```python
from build123d import *

# Parameters (mm, degrees)
F0_R     = 1.25
F1_DEPTH = 5
F2_DEPTH = 6
F3_R     = 3.5
F4_DEPTH = 2
F5_R     = 3.5
F6_DEPTH = 2
F7_R     = 0.99999


# Not quite as in the source:
# - a fillet or chamfer is up to 0.001 mm smaller than in the source, because OpenCascade refuses the exact size


with BuildPart() as f1:
    # F0 (on Top) → F1 (new body)
    with BuildSketch(Plane.XY):
        with BuildLine():
            ThreePointArc((-24.6972243623, -3), (-23.4537141687, -1.7234101758), (-23, 0))
            ThreePointArc((-23, 0), (-23.4537141687, 1.7234101758), (-24.6972243623, 3))
            ThreePointArc((-24.6972243623, 3), (-30, 0), (-24.6972243623, -3))
        make_face()
        with Locations((-26.5, 0)):
            Circle(F0_R, mode=Mode.SUBTRACT)
    extrude(amount=F1_DEPTH)



with BuildPart() as f1b:
    # F0 (on Top) → F1, piece 2 (new body)
    with BuildSketch(Plane.XY):
        with BuildLine():
            ThreePointArc((30, 0), (28.2234101758, 3.0462858313), (24.6972243623, 3))
            ThreePointArc((24.6972243623, 3), (23, 0), (24.6972243623, -3))
            ThreePointArc((24.6972243623, -3), (28.2234101758, -3.0462858313), (30, 0))
        make_face()
        with Locations((26.5, 0)):
            Circle(F0_R, mode=Mode.SUBTRACT)
    extrude(amount=F1_DEPTH)


with BuildPart() as f1_1:
    add(f1.part)

    add(f1b.part)  # F2 merges F1b
    # F0 (on Top) → F2 (join)
    with BuildSketch(Plane.XY):
        with BuildLine():
            ThreePointArc((-24.6972243623, 3), (-23.4537141687, 1.7234101758), (-23, 0))
            ThreePointArc((-23, 0), (-23.4537141687, -1.7234101758), (-24.6972243623, -3))
            Line((-24.6972243623, -3), (24.6972243623, -3))
            ThreePointArc((24.6972243623, -3), (23, 0), (24.6972243623, 3))
            Line((24.6972243623, 3), (-24.6972243623, 3))
        make_face()
    extrude(amount=F2_DEPTH)

    # F3 (on face) → F4 (join)
    with BuildSketch(Plane.XY.offset(5)):
        with Locations((-26.5, 0)):
            Circle(F3_R)
    extrude(amount=F4_DEPTH)

    # F5 (on face) → F6 (join)
    with BuildSketch(Plane.XY.offset(5)):
        with Locations((26.5, 0)):
            Circle(F5_R)
    extrude(amount=F6_DEPTH)

    # F7 (radius 1 in the source; OpenCascade refuses exactly that, so slightly less here)
    f7_edges = [f1_1.edges().sort_by_distance(p)[0] for p in [
        (0, 3, 6),
        (0, -3, 6),
        (23, 0, 7),
        (-30, 0, 7),
    ]]
    fillet(f7_edges, radius=F7_R)


solid = f1_1.part
```
CAD build for the part. Positions are in the model's coordinates, mm. A direction names the side the tool comes from. Give positions to 0.01 mm unless a question says otherwise; leave off trailing zeros. Order: outer loops, then holes, each group sorted by start corner. A loop starts at its lowest first (then second) coordinate and runs counter-clockwise, first axis right, second up. Notation, with made-up numbers: M 71,-4 L 101,-4 A29 cw 101,29 Z; hole C -5.75,-25 d4. An arc over 180 degrees is marked long. Put each result on its own line as item: value. Start each with the question number.
(1) Saw through at A-A, the plane x = -26.5. Write the cut outline in (y, z).
(2) Flat gauge pins, fed straight in: pin 1 Ø1.5 at (y, z) = (2.5, 1.5) entering from -X; pin 2 Ø0.8 at (x, y) = (27, 0.5) entering from -Z; pin 3 Ø1.5 at (x, z) = (-14, 3.5) entering from +Y. Where does each tip first touch, or does it go through?
(3) Drill centre lines: line 1 along Y through (x, z) = (-26.5, 1.5); line 2 along Z through (x, y) = (0, 1.25); line 3 along Y through (x, z) = (14.5, 3.25). Where is each one in solid material? Low to high.
(4) Saw through at B-B, the plane z = 3.75. Write the cut outline in (x, y).
(5) Which spindle directions (+Z, -Z, +X, -X, +Y, -Y) get a long thin tool onto all of the face, cutting with end or side? Do faces 4 (the cylindrical face through (-25.345, -0.479, 2.465)), 5 (the flat face through (0, 3, 2)), 6 (the flat face through (-27, 0, 7)), 7 (the cylindrical face through (0.346, -2.699, 5.715)), 8 (the flat face through (0, -3, 2)). Say none if no direction does.
(6) Mould opens along X. For faces 1 (the flat face through (26, 0, 5)), 2 (the flat face through (0, 0, 0)), 3 (the cylindrical face through (-0.346, 2.715, 5.699)) say: +X half, -X half, draft (parallel to the pull), parting line (faces both ways), or undercut.
Check result:
1. outline: M -3.5,0 L -1.25,0 L -1.25,5 L 1.25,5 L 1.25,0 L 3.5,0 L 3.5,6 A1 ccw 2.5,7 L -2.5,7 A1 ccw -3.5,6 Z
2. pin 1: stops at x = -29.53
2. pin 2: stops at z = 5
2. pin 3: stops at y = 3
3. line 1: y = -3.5 to -1.25, 1.25 to 3.5
3. line 2: z = 0 to 6
3. line 3: y = -3 to 3
4. outline: M -24.7,-3 L 24.7,-3 A3.5 ccw long 24.7,3 L -24.7,3 A3.5 ccw long Z; hole C -26.5,0 d2.5; hole C 26.5,0 d2.5
5. face 4: -Z
5. face 5: +Z, -Z, +Y
5. face 6: +Z, +X, -X, +Y, -Y
5. face 7: +Z, -Y
5. face 8: +Z, -Z, -Y
6. face 1: undercut
6. face 2: draft
6. face 3: undercut
